```python
from build123d import *

# Parameters (mm, degrees)
SKETCH1_W           = 260
SKETCH1_H           = 100
BOSS_EXTRUDE1_DEPTH = 10
SKETCH3_W           = 55
SKETCH3_H           = 10
SKETCH3_W_2         = 60
SKETCH3_W_3         = 45
CUT_EXTRUDE2_DEPTH  = 140.642400438
FILLET1_R           = 2
SKETCH2_R           = 6.25
CUT_EXTRUDE1_DEPTH  = 140.642400438
CHAMFER1_SIZE       = 2
SKETCH4_R           = 2.3
CUT_EXTRUDE3_DEPTH  = 6.2


with BuildPart() as part:
    # Sketch1 → Boss-Extrude1 (new body)
    with BuildSketch(Plane(origin=(0, 0, 0), x_dir=(1, 0, 0), z_dir=(0, 1, 0))):
        Rectangle(SKETCH1_W, SKETCH1_H)
    extrude(amount=BOSS_EXTRUDE1_DEPTH)

    # Sketch3 → Cut-Extrude2 (cut, through all)
    with BuildSketch(Plane(origin=(0, 10, 0), x_dir=(1, 0, 0), z_dir=(0, 1, 0))):
        with Locations((102.5, 45)):
            Rectangle(SKETCH3_W, SKETCH3_H)
        with Locations((102.5, -45)):
            Rectangle(SKETCH3_W, SKETCH3_H)
        Polygon((-130, -50), (-30, -50), (-30, -40), (-120, -40), (-120, 50), (-130, 50), (-130, -40), align=None)
        with Locations((-60, 45)):
            Rectangle(SKETCH3_W_2, SKETCH3_H)
        with Locations((22.5, 45)):
            Rectangle(SKETCH3_W_3, SKETCH3_H)
        with Locations((22.5, -45)):
            Rectangle(SKETCH3_W_3, SKETCH3_H)
    extrude(amount=-CUT_EXTRUDE2_DEPTH, mode=Mode.SUBTRACT)

    # Fillet1
    fillet1_edges = [part.edges().sort_by_distance(p)[0] for p in [
        (-15, 10, 50),
        (60, 10, 50),
        (130, 10, 0),
        (60, 10, -50),
        (-15, 10, -50),
        (-105, 10, -50),
        (0, 10, -45),
        (22.5, 10, -40),
        (45, 10, -45),
        (-90, 10, -45),
        (-60, 10, -40),
        (-30, 10, -45),
        (-30, 10, 45),
        (-75, 10, 40),
        (-120, 10, -5),
        (102.5, 10, 40),
        (75, 10, 45),
        (0, 10, 45),
        (45, 10, 45),
        (22.5, 10, 40),
        (75, 10, -45),
        (102.5, 10, -40),
    ]]
    fillet(fillet1_edges, radius=FILLET1_R)

    # Sketch2 → Cut-Extrude1 (cut, through all)
    with BuildSketch(Plane(origin=(0, 10, 0), x_dir=(1, 0, 0), z_dir=(0, 1, 0))):
        with Locations(Location((-105, 0, 0), (0, 0, 270))):
            Circle(SKETCH2_R)
    extrude(amount=-CUT_EXTRUDE1_DEPTH, mode=Mode.SUBTRACT)

    # Chamfer1
    chamfer1_edges = [part.edges().sort_by_distance(p)[0] for p in [
        (-105, 10, -6.25),
    ]]
    chamfer(chamfer1_edges, length=CHAMFER1_SIZE)

    # Sketch4 → Cut-Extrude3 (cut)
    with BuildSketch(Plane(origin=(0, 10, 0), x_dir=(1, 0, 0), z_dir=(0, 1, 0))):
        with Locations(Location((59.5, 39, 0), (0, 0, 270))):
            Circle(SKETCH4_R)
        with Locations(Location((-14.5, 39, 0), (0, 0, 270))):
            Circle(SKETCH4_R)
        with Locations(Location((59.5, -39, 0), (0, 0, 270))):
            Circle(SKETCH4_R)
        with Locations(Location((-14.5, -39, 0), (0, 0, 270))):
            Circle(SKETCH4_R)
    extrude(amount=-CUT_EXTRUDE3_DEPTH, mode=Mode.SUBTRACT)


solid = part.part
```
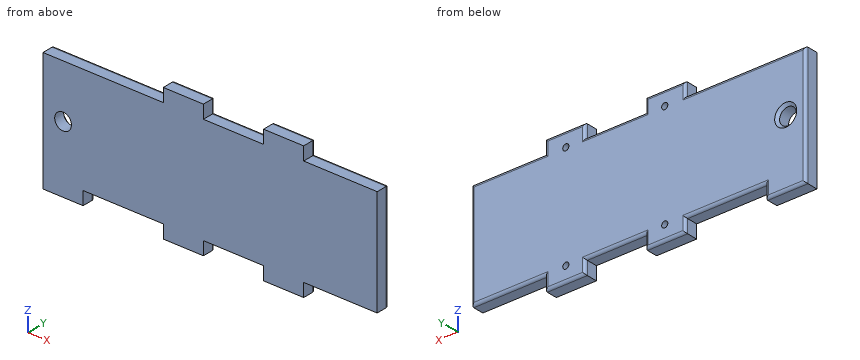
Geometry: final body of the model. Coordinates: model frame, mm. Give positions to 0.01 mm unless a question says otherwise; leave off trailing zeros. Loops run counter-clockwise (first coordinate to the right, second up) from the corner with the lowest first, then second, coordinate; pieces in that order, holes last. Notation, with made-up numbers: (4, -6.75) -> (54, -6.75) arc R14 ccw to (54, 4.25) -> close; hole circle Ø6 at (27.5, 8). An arc over 180 degrees is marked (long way). Return JSON: item names as keys, results as strings.
Item 1: Line query: line 1 (X direction, y = 6.5, z = -39); line 2 (X direction, y = 6.5, z = 43); line 3 (Z direction, x = 102, y = 6.25). Output: solid intervals per line, ascending.
Filled in:
{"line 1": "-120 to -16.8, -12.2 to 57.2, 61.8 to 130", "line 2": "-30 to 0, 45 to 75", "line 3": "-40 to 40"}
Item 2: Section B-B, the plane x = -105. Output: boundary loops of the cut face in (y, z).
Filled in:
{"outline": "(0, -50) -> (8, -50) arc R2 ccw to (10, -48) -> (10, -8.25) -> (8, -6.25) -> (0, -6.25) -> close; (0, 6.25) -> (8, 6.25) -> (10, 8.25) -> (10, 38) arc R2 ccw to (8, 40) -> (0, 40) -> close"}
Item 3: Section A-A, the plane y = 2. Output: boundary loops of the cut face in (x, z).
Filled in:
{"outline": "(-120, -50) -> (-90, -50) -> (-90, -40) -> (-30, -40) -> (-30, -50) -> (0, -50) -> (0, -40) -> (45, -40) -> (45, -50) -> (75, -50) -> (75, -40) -> (130, -40) -> (130, 40) -> (75, 40) -> (75, 50) -> (45, 50) -> (45, 40) -> (0, 40) -> (0, 50) -> (-30, 50) -> (-30, 40) -> (-120, 40) -> close; hole circle Ø12.5 at (-105, 0)"}
Item 4: Section D-D, the plane x = -52.5. Output: boundary loops of the cut face in (y, z), plus the area to 3 significant figures.
Filled in:
{"outline": "(0, -40) -> (8, -40) arc R2 ccw to (10, -38) -> (10, 38) arc R2 ccw to (8, 40) -> (0, 40) -> close", "area": "798 mm^2"}
Item 5: Section C-C, the plane x = -14.5. Output: boundary loops of the cut face in (y, z), plus the area to 3 significant figures.
Filled in:
{"outline": "(0, -50) -> (8, -50) arc R2 ccw to (10, -48) -> (10, -41.3) -> (3.8, -41.3) -> (3.8, -36.7) -> (10, -36.7) -> (10, 36.7) -> (3.8, 36.7) -> (3.8, 41.3) -> (10, 41.3) -> (10, 48) arc R2 ccw to (8, 50) -> (0, 50) -> close", "area": "941 mm^2"}
Item 6: Pin query (flat end, axial travel): P1, Ø5.5, axis at x = -14.5, z = -39, coming from the -Y side; P2, Ø2.5, axis at x = -14.5, z = -39.5, coming from the +Y side; P3, Ø2.5, axis at y = 4.5, z = 46, coming from the -X side; P4, Ø3, axis at x = 6, y = 4, coming from the -Z side. Return the tip coordinate at first contact, or that it passes through.
Filled in:
{"P1": "y = 0", "P2": "y = 3.8", "P3": "x = -30", "P4": "z = -40"}
